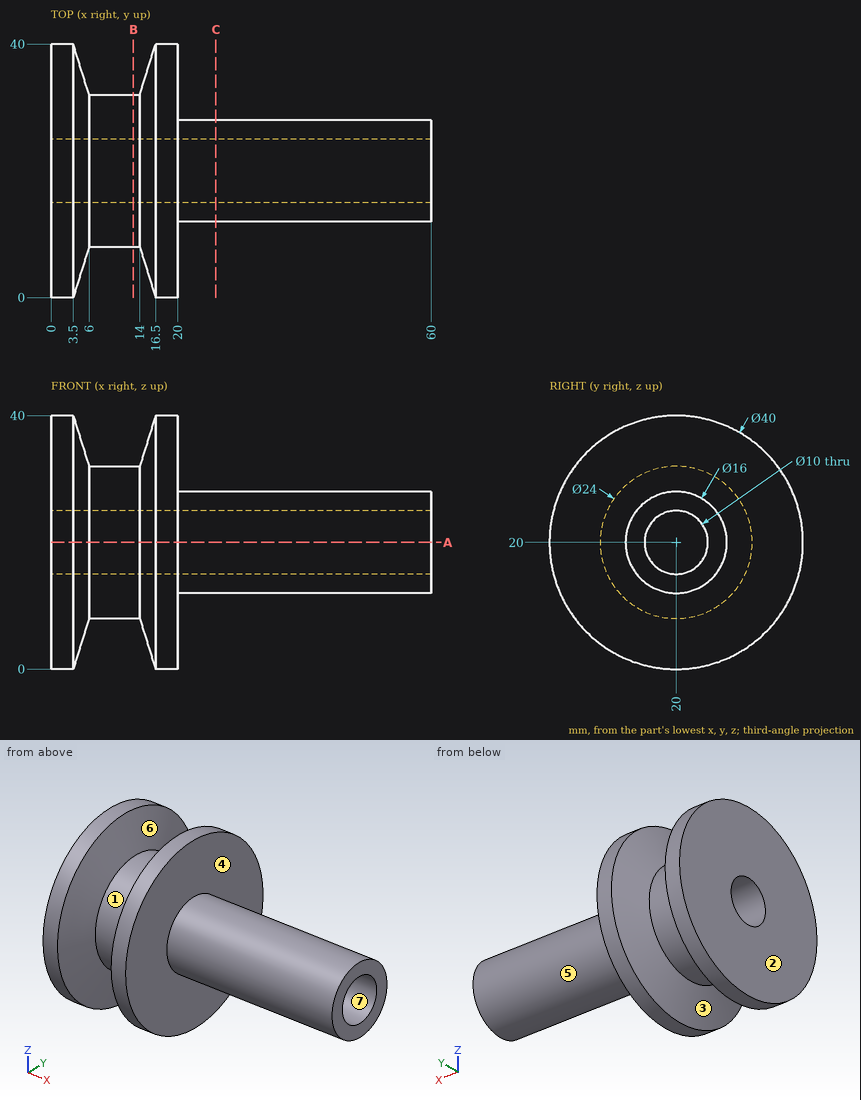
Source: three-view drawing plus pictorial views. Frame: mm from the lowest corner of the part. A direction names the side the tool comes from. Round coordinates to 2 decimals unless told otherwise and drop trailing zeros. Loops run counter-clockwise (first coordinate to the right, second up) from the corner with the lowest first, then second, coordinate; pieces in that order, holes last. Notation, with made-up numbers: (-26.5, 86) -> (-13.5, 86) arc R28 ccw to (-13.5, 108) -> close; hole circle Ø10 at (74, 50). An arc over 180 degrees is marked (long way). Use one line per item in the form item = value.
Item 1: Material intervals for probe 1 along Z at (x, y) = (23, 20); probe 2 along Z at (x, y) = (17, 20); probe 3 along X at (y, z) = (18.5, 9.5), sorted ascending.
Evaluation:
probe_1 = 12 to 15, 25 to 28
probe_2 = 0 to 15, 25 to 40
probe_3 = 0 to 20
Item 2: Cut plane A-A on z = 20. Output: boundary loops of the cut face in (x, y), then the cut area to 3 significant figures.
Evaluation:
outline = (0, 0) -> (3.5, 0) -> (6, 8) -> (14, 8) -> (16.5, 0) -> (20, 0) -> (20, 12) -> (60, 12) -> (60, 15) -> (0, 15) -> close; (0, 25) -> (60, 25) -> (60, 28) -> (20, 28) -> (20, 40) -> (16.5, 40) -> (14, 32) -> (6, 32) -> (3.5, 40) -> (0, 40) -> close
area = 672 mm2
Item 3: Cut plane B-B on x = 13. Output: boundary loops of the cut face in (y, z).
Evaluation:
outline = circle Ø24 at (20, 20); hole circle Ø10 at (20, 20)
Item 4: Cut plane C-C on x = 26. Output: boundary loops of the cut face in (y, z), then the cut area to 3 significant figures.
Evaluation:
outline = circle Ø16 at (20, 20); hole circle Ø10 at (20, 20)
area = 123 mm2
Item 5: Draft query along X for the marked faces 1, 2, 3 and 4. Return one class per face: released by +X, released by -X, zero draft, split by the parting line, or undercut.
Evaluation:
face_1 = undercut
face_2 = released by -X
face_3 = undercut
face_4 = released by +X
Item 6: Access query for the marked faces 5, 6 and 7. Directions: +Z, -Z, +X, -X, +Y, -Y. A direction counts if a zero-diameter tool reaches every point of the face in a straight line with its end or side. Return the directions, or none.
Evaluation:
face_5 = +X
face_6 = none
face_7 = +X, -X
Item 7: Contact query for flat-ended pins moving along their axis: pin 1 Ø1 at (x, y) = (9, 12.5) entering from -Z; pin 2 Ø12 at (x, y) = (18, 11.5) entering from -Z; pin 3 Ø2 at (x, y) = (31.5, 15) entering from -Z. Output: stop coordinate, or through.
Evaluation:
pin_1 = 10.25
pin_2 = 0.16
pin_3 = 13.07
